from build123d import *

# Parameters (mm, degrees)
F0_W     = 20
F0_H     = 55
F0_R     = 1.6
F1_DEPTH = 3.2
F2_DEPTH = 3.2
F3_DEPTH = 3.2


with BuildPart() as f1:
    # F0 (on Top) → F1 (new body)
    with BuildSketch(Plane.XY):
        Rectangle(F0_W, F0_H)
        with Locations((0, -19.831753)):
            Circle(F0_R, mode=Mode.SUBTRACT)
        with Locations((-4.759501, 22.12626)):
            Circle(F0_R, mode=Mode.SUBTRACT)
        with Locations((5.231229, 21.486786)):
            Circle(F0_R, mode=Mode.SUBTRACT)
    extrude(amount=F1_DEPTH)

    # F0 (on Top) → F2 (join)
    with BuildSketch(Plane.XY):
        Rectangle(F0_W, F0_H)
        with Locations((0, -19.831753)):
            Circle(F0_R, mode=Mode.SUBTRACT)
        with Locations((-4.759501, 22.12626)):
            Circle(F0_R, mode=Mode.SUBTRACT)
        with Locations((5.231229, 21.486786)):
            Circle(F0_R, mode=Mode.SUBTRACT)
    extrude(amount=F2_DEPTH)

    # F0 (on Top) → F3 (join)
    with BuildSketch(Plane.XY):
        Rectangle(F0_W, F0_H)
        with Locations((0, -19.831753)):
            Circle(F0_R, mode=Mode.SUBTRACT)
        with Locations((-4.759501, 22.12626)):
            Circle(F0_R, mode=Mode.SUBTRACT)
        with Locations((5.231229, 21.486786)):
            Circle(F0_R, mode=Mode.SUBTRACT)
    extrude(amount=F3_DEPTH)


solid = f1.part
Read the model definition and answer for the solid it produces. Units are mm, in the model's axes. Round coordinates to 2 decimals unless told otherwise and drop trailing zeros. Order: outer loops, then holes, each group sorted by start corner. A loop starts at its lowest first (then second) coordinate and runs counter-clockwise, first axis right, second up.
1) The part is cut by section B-B on z = 1.95. Write down the section's boundary in (x, y), plus the area to 3 significant figures.
2) Straight lines are drawn through the part: L1, parallel to Y at x = 0, z = 0.8; L2, parallel to X at y = -19, z = 0.8; L3, parallel to Y at x = -5, z = 0.4. For each, find the intervals that lie inside material, in ascending order.
3) The mould has two halves that part along X. Classify faces 1 (the face through (-4.968, 23.713, 1.578)), 2 (the face through (3.962, 20.513, 1.578)), 3 (the face through (0, 0, 3.2)), 4 (the face through (10, 0, 2)): released by +X, released by -X, zero draft, split by the parting line, or undercut.
4) The part is cut by section C-C on x = 6. Write down the section's boundary in (y, z).
5) A flat-ended cylindrical pin translates along its axis: pin 1 (2.5 mm diameter, centred on x = 5.23, y = 21.49, fed in from +Z). Find the tip coordinate at first contact, or state that the pin passes through.
6) The part is cut by section A-A on x = 0. Write down the section's boundary in (y, z), plus the area to 3 significant figures.
Resolved:
1. outline: (-10, -27.5) - (10, -27.5) - (10, 27.5) - (-10, 27.5) - close; hole circle Ø3.2 at (-4.76, 22.13); hole circle Ø3.2 at (0, -19.83); hole circle Ø3.2 at (5.23, 21.49)
1. area: 1,080 mm2
2. L1: y = -27.5 to -21.43, -18.23 to 27.5
2. L2: x = -10 to -1.37, 1.37 to 10
2. L3: y = -27.5 to 20.54, 23.71 to 27.5
3. face 1: undercut
3. face 2: undercut
3. face 3: zero draft
3. face 4: released by +X
4. outline: (-27.5, 0) - (20.08, 0) - (20.08, 3.2) - (-27.5, 3.2) - close; (22.89, 0) - (27.5, 0) - (27.5, 3.2) - (22.89, 3.2) - close
5. pin 1: passes through
6. outline: (-27.5, 0) - (-21.43, 0) - (-21.43, 3.2) - (-27.5, 3.2) - close; (-18.23, 0) - (27.5, 0) - (27.5, 3.2) - (-18.23, 3.2) - close
6. area: 166 mm2
